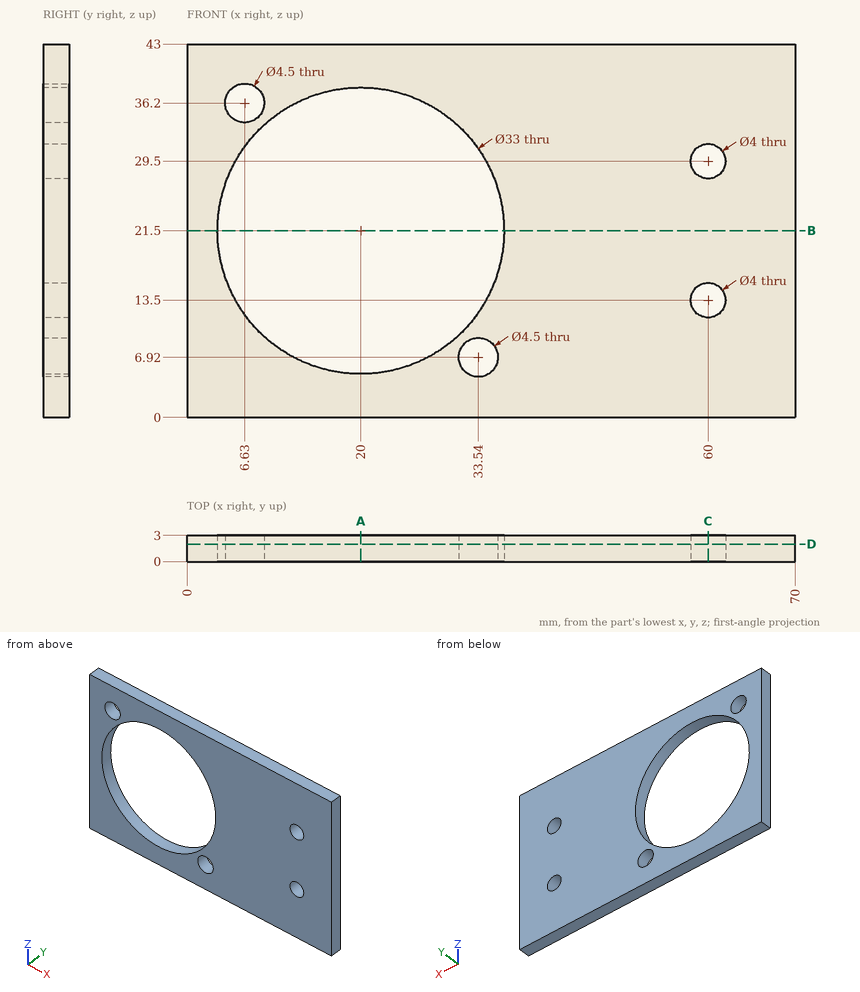
Geometry: see drawing. Coordinates: mm, zero at the bounding-box minimum. Round coordinates to 2 decimals unless told otherwise and drop trailing zeros. Loops run counter-clockwise (first coordinate to the right, second up) from the corner with the lowest first, then second, coordinate; pieces in that order, holes last. Notation, with made-up numbers: M 22,29.5 L 70,29.5 A18 ccw 70,38.5 Z; hole C -5,29.5 d3. An arc over 180 degrees is marked long. Use a Markdown table: item, result. Add a question column.
1. Section query B-B on z = 21.5. Return the cut outline in (x, y), then the cut area to 3 significant figures.
2. Section query A-A on x = 20. Return the cut outline in (y, z), then the cut area to 3 significant figures.
3. Section query D-D on y = 2. Return the cut outline in (x, z).
4. Line query: line 1 (Z direction, x = 33, y = 1.4); line 2 (X direction, y = 1.15, z = 21.5); line 3 (X direction, y = 0.1, z = 13.5). Output: solid intervals per line, ascending.
5. Section query C-C on x = 60. Return the cut outline in (y, z).
6. Contact query for a flat-ended pin moving along its axis: P1, Ø4, axis at x = 33.54, z = 6.92, coming from the +Y side. Output: stop coordinate, or through.
Reported:
| question | item | result |
|---|---|---|
| 1 | outline | M 0,0 L 3.5,0 L 3.5,3 L 0,3 Z; M 36.5,0 L 70,0 L 70,3 L 36.5,3 Z |
| 1 | area | 111 mm² |
| 2 | outline | M 0,0 L 3,0 L 3,5 L 0,5 Z; M 0,38 L 3,38 L 3,43 L 0,43 Z |
| 2 | area | 30.0 mm² |
| 3 | outline | M 0,0 L 70,0 L 70,43 L 0,43 Z; hole C 20,21.5 d33; hole C 6.63,36.2 d4.5; hole C 33.54,6.92 d4.5; hole C 60,13.5 d4; hole C 60,29.5 d4 |
| 4 | line 1 | z = 0 to 4.74, 9.1 to 11.34, 31.66 to 43 |
| 4 | line 2 | x = 0 to 3.5, 36.5 to 70 |
| 4 | line 3 | x = 0 to 5.57, 34.43 to 58, 62 to 70 |
| 5 | outline | M 0,0 L 3,0 L 3,11.5 L 0,11.5 Z; M 0,15.5 L 3,15.5 L 3,27.5 L 0,27.5 Z; M 0,31.5 L 3,31.5 L 3,43 L 0,43 Z |
| 6 | P1 | passes through |
